from build123d import *

# Parameters (mm, degrees)
SKETCH3_R          = 35
CUT_EXTRUDE2_DEPTH = 285
CUT_EXTRUDE3_DEPTH = 197


with BuildPart() as part:
    # Loft1: read off the stored shape, not the designer's step
    # Loft1: loft between two sections, ruled curve by curve
    loft1_from = [
        Edge.make_bspline([(-87.451090027, 6.495669107, 0), (-100.442428241, -168.406510946, 0), (74.459751812, -181.397849161, 0), (87.451090027, -6.495669107, 0), (100.442428241, 168.406510946, 0), (-74.459751812, 181.397849161, 0), (-87.451090027, 6.495669107, 0)], [0, 0, 0, 0, 0.5, 0.5, 0.5, 1, 1, 1, 1], 3, [1, 0.333333333, 0.333333333, 1, 0.333333333, 0.333333333, 1]),
    ]
    loft1_to = [
        Edge.make_bspline([(-125.095140395, -21.913599651, 200), (-81.267941093, -272.10388044, 200), (168.922339696, -228.276681139, 200), (125.095140395, 21.913599651, 200), (81.267941093, 272.10388044, 200), (-168.922339696, 228.276681139, 200), (-125.095140395, -21.913599651, 200)], [0, 0, 0, 0, 0.5, 0.5, 0.5, 1, 1, 1, 1], 3, [1, 0.333333333, 0.333333333, 1, 0.333333333, 0.333333333, 1]),
    ]
    loft1 = Solid(Shell([*[Face.make_surface_from_curves(loft1_from[k], loft1_to[k]) for k in range(1)], Face(Wire(loft1_from)), Face(Wire(loft1_to))]))
    add(loft1)

    # Sketch3 → Cut-Extrude2 (cut)
    with BuildSketch(Plane.XY.offset(200)):
        Circle(SKETCH3_R)
        with BuildLine():
            ThreePointArc((-17.5, -30.310889132), (-33.80740392, 9.058666579), (0, 35))
            Line((0, 35), (0, 127))
            ThreePointArc((0, 127), (-97.242036064, 81.688349366), (-125.095140395, -21.913599651))
            ThreePointArc((-125.095140395, -21.913599651), (-104.072977278, -72.786093456), (-63.5, -109.985226281))
            Line((-63.5, -109.985226281), (-17.5, -30.310889132))
        make_face()
    extrude(amount=-CUT_EXTRUDE2_DEPTH, mode=Mode.SUBTRACT)

    # Sketch4 → Cut-Extrude3 (cut)
    with BuildSketch(Plane.XY.offset(200)):
        with BuildLine():
            Line((0, 127), (0, 35))
            ThreePointArc((0, 35), (19.456058328, 29.09401647), (32.345993225, 13.36924539))
            Line((32.345993225, 13.36924539), (118.819608286, 44.843067322))
            ThreePointArc((118.819608286, 44.843067322), (72.228562391, 104.460685308), (0, 127))
        make_face()
        with BuildLine():
            Line((119.845668716, 42.02398946), (33.372053655, 10.550167528))
            ThreePointArc((33.372053655, 10.550167528), (33.80740392, -9.058666579), (23.625962477, -25.822739921))
            Line((23.625962477, -25.822739921), (82.777398912, -96.316676798))
            ThreePointArc((82.777398912, -96.316676798), (122.672579939, -32.870018728), (119.845668716, 42.02398946))
        make_face()
        with BuildLine():
            Line((80.479265582, -98.245039627), (21.327829148, -27.75110275))
            ThreePointArc((21.327829148, -27.75110275), (2.302432535, -34.924186525), (-17.5, -30.310889132))
            Line((-17.5, -30.310889132), (-63.5, -109.985226281))
            ThreePointArc((-63.5, -109.985226281), (10.321427256, -126.579888369), (80.479265582, -98.245039627))
        make_face()
    extrude(amount=-CUT_EXTRUDE3_DEPTH, mode=Mode.SUBTRACT)


solid = part.part
The model under review builds one solid part; all positions refer to its coordinate system, in mm. A direction names the side the tool comes from. Round coordinates to 2 decimals unless told otherwise and drop trailing zeros. Write item = value, one per line. Start each with the question number.
Item 1: To check wall thickness, follow L1, parallel to Z at x = 57, y = -26; L2, parallel to Y at x = 98, z = 94; L3, parallel to Y at x = 49.5, z = 19. State the ranges of each line that lie inside material, in increasing order.
Item 2: Insertion check: pin 1 (4 mm diameter, centred on x = 18, y = 59.5, fed in from +Z); pin 2 (3.5 mm diameter, centred on y = 60.5, z = 1, fed in from -X); pin 3 (10 mm diameter, centred on y = 6, z = 70, fed in from -X). Each pin has a flat end and moves straight along its axis. Give the tip position at first contact, or say it passes through.
Item 3: Mouldability with a two-part tool opening along Y and no side actions: class faces 1 (the flat face through (46.215, -52.744, 102.879)), 2 (the flat face through (44.745, -55.659, 102.879)), 3 (the flat face through (38, -13, 0)) as released by +Y, released by -Y, zero draft, split by the parting line, or undercut.
Item 4: For faces 4 (the flat face through (5, -64, 3)), 5 (the flat face through (67.61, 23.01, 102.88)), 6 (the flat face through (52, -62, 200)), 7 (the flat face through (-30.99, -53.68, 1.52)), 8 (the flat face through (65.4, 25.4, 102.9)), list the 3-axis set-ups (+Z, -Z, +X, -X, +Y, -Y) from which the entire face can be reached by the end or side of a thin tool; tool diameter is ignored.
Result:
q1.L1 = 0 to 3
q1.L2 = 34.07 to 37.27
q1.L3 = -61.33 to -56.66, 16.42 to 19.61
q2.pin_1 = 3
q2.pin_2 = 0
q2.pin_3 = 33.23
q3.face_1 = undercut
q3.face_2 = released by -Y
q3.face_3 = zero draft
q4.face_4 = +Z, -X, -Y
q4.face_5 = +Z, +X
q4.face_6 = +Z, +X, -X, +Y, -Y
q4.face_7 = +Z, -Z, -X, +Y
q4.face_8 = +Z, -X, +Y
